The listing builds one solid part. Answer for the finished solid, in the listing's coordinates (mm). Face numbers are marked on the shaded views. A direction names the side the tool comes from. Give positions to 0.01 mm unless a question says otherwise; leave off trailing zeros. Write each loop counter-clockwise with the first axis right and the second up, starting at its lowest first coordinate (ties: lowest second). Pieces come first, ordered by that corner, then holes.
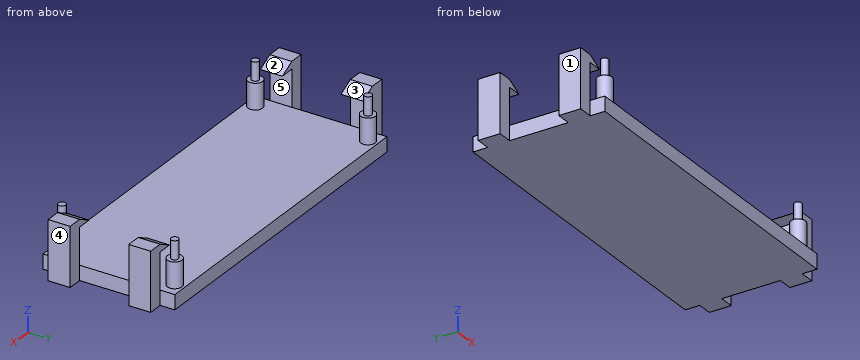
```python
from build123d import *

# Parameters (mm, degrees)
F0_R     = 1
F0_R_2   = 0.5
F1_DEPTH = 2
F2_DEPTH = 5.5
F3_DEPTH = 8
F0_W     = 2
F0_H     = 3
F4_DEPTH = 8
F6_DEPTH = 3


# Not quite as in the source:
# - a feature names something its author has since deleted; it is built from what else it names


with BuildPart() as f1:
    # F0 (on Top) → F1 (new body)
    with BuildSketch(Plane.XY):
        Polygon((22.5, 9), (-22.5, 9), (-22.5, 7), (-22.5, 4), (-22.5, -4), (-22.5, -7), (-22.5, -9), (22.5, -9), (22.5, -7), (22.5, -4), (22.5, 4), (22.5, 7), align=None)
        with Locations((-20.5, -7.7)):
            Circle(F0_R, mode=Mode.SUBTRACT)
        with Locations((20.5, -7.7)):
            Circle(F0_R, mode=Mode.SUBTRACT)
        with Locations((-20.5, 7.7)):
            Circle(F0_R, mode=Mode.SUBTRACT)
        with Locations((20.5, 7.7)):
            Circle(F0_R, mode=Mode.SUBTRACT)
        with Locations((-20.5, 7.7)):
            Circle(F0_R)
        with Locations((-20.5, 7.7)):
            Circle(F0_R_2, mode=Mode.SUBTRACT)
        with Locations((20.5, 7.7)):
            Circle(F0_R)
        with Locations((20.5, 7.7)):
            Circle(F0_R_2, mode=Mode.SUBTRACT)
        with Locations((20.5, -7.7)):
            Circle(F0_R)
        with Locations((20.5, -7.7)):
            Circle(F0_R_2, mode=Mode.SUBTRACT)
        with Locations((-20.5, -7.7)):
            Circle(F0_R)
        with Locations((-20.5, -7.7)):
            Circle(F0_R_2, mode=Mode.SUBTRACT)
        with Locations((-20.5, 7.7)):
            Circle(F0_R_2)
        with Locations((20.5, 7.7)):
            Circle(F0_R_2)
        with Locations((20.5, -7.7)):
            Circle(F0_R_2)
        with Locations((-20.5, -7.7)):
            Circle(F0_R_2)
    extrude(amount=F1_DEPTH)

    # F0 (on Top) → F2 (join)
    with BuildSketch(Plane.XY):
        with Locations((-20.5, 7.7)):
            Circle(F0_R)
        with Locations((-20.5, 7.7)):
            Circle(F0_R_2, mode=Mode.SUBTRACT)
        with Locations((-20.5, 7.7)):
            Circle(F0_R_2)
        with Locations((-20.5, -7.7)):
            Circle(F0_R)
        with Locations((-20.5, -7.7)):
            Circle(F0_R_2, mode=Mode.SUBTRACT)
        with Locations((-20.5, -7.7)):
            Circle(F0_R_2)
        with Locations((20.5, 7.7)):
            Circle(F0_R)
        with Locations((20.5, 7.7)):
            Circle(F0_R_2, mode=Mode.SUBTRACT)
        with Locations((20.5, 7.7)):
            Circle(F0_R_2)
        with Locations((20.5, -7.7)):
            Circle(F0_R)
        with Locations((20.5, -7.7)):
            Circle(F0_R_2, mode=Mode.SUBTRACT)
        with Locations((20.5, -7.7)):
            Circle(F0_R_2)
    extrude(amount=F2_DEPTH)

    # F0 (on Top) → F3 (join)
    with BuildSketch(Plane.XY):
        with Locations((-20.5, 7.7)):
            Circle(F0_R_2)
        with Locations((20.5, 7.7)):
            Circle(F0_R_2)
        with Locations((20.5, -7.7)):
            Circle(F0_R_2)
        with Locations((-20.5, -7.7)):
            Circle(F0_R_2)
    extrude(amount=F3_DEPTH)

    # F0 (on Top) → F4 (join)
    with BuildSketch(Plane.XY):
        with Locations((-23.5, 5.5)):
            Rectangle(F0_W, F0_H)
    extrude(amount=F4_DEPTH)

    # F5 (on face) → F6 (join, through all)
    with BuildSketch(Plane.XZ.offset(-4)):
        Polygon((-22.5, 8), (-22.5, 6.980669219), (-20.5, 6.980669219), align=None)
    extrude(amount=-F6_DEPTH)

    # F7: F1 across plane


with BuildPart() as f1_1:
    add(f1.part)
    add(f1.part.mirror(Plane.XZ))

    # F8: F1 across plane


with BuildPart() as f1_2:
    add(f1_1.part)
    add(f1_1.part.mirror(Plane.YZ))


solid = f1_2.part
```
Item 1: Which of the six approach directions +Z, -Z, +X, -X, +Y, -Y give full straight-line access (tool end or side, diameter ignored) to the marked faces 1 and 2?
Conclusion:
face 1: +Z, -Z, -X, +Y, -Y
face 2: +Z
Item 2: A cutting plane is placed at A-A, the plane y = -7.7. Give the vertices of the cut face in (x, z).
Conclusion:
outline: (-22.5, 0) - (22.5, 0) - (22.5, 2) - (21.5, 2) - (21.5, 5.5) - (21, 5.5) - (21, 8) - (20, 8) - (20, 5.5) - (19.5, 5.5) - (19.5, 2) - (-19.5, 2) - (-19.5, 5.5) - (-20, 5.5) - (-20, 8) - (-21, 8) - (-21, 5.5) - (-21.5, 5.5) - (-21.5, 2) - (-22.5, 2) - close
Item 3: A cutting plane is placed at C-C, the plane x = 16.5. Give the vertices of the cut face in (y, z), plus the area to 3 significant figures.
Conclusion:
outline: (-9, 0) - (9, 0) - (9, 2) - (-9, 2) - close
area: 36.0 mm2
Item 4: Consider probe 1 along X at (y, z) = (-6.5, 2.75); probe 2 along Z at (x, y) = (-11.5, -3); probe 3 along X at (y, z) = (-8, 5.75). Determine where each line is inside the solid, lowest interval first.
Conclusion:
probe 1: x = -24.5 to -22.5, 22.5 to 24.5
probe 2: z = 0 to 2
probe 3: x = -20.9 to -20.1, 20.1 to 20.9
Item 5: A cutting plane is placed at B-B, the plane z = 1.25. Give the vertices of the cut face in (x, y), plus the area to 3 significant figures.
Conclusion:
outline: (-24.5, -7) - (-22.5, -7) - (-22.5, -9) - (22.5, -9) - (22.5, -7) - (24.5, -7) - (24.5, -4) - (22.5, -4) - (22.5, 4) - (24.5, 4) - (24.5, 7) - (22.5, 7) - (22.5, 9) - (-22.5, 9) - (-22.5, 7) - (-24.5, 7) - (-24.5, 4) - (-22.5, 4) - (-22.5, -4) - (-24.5, -4) - close
area: 834 mm2
Item 6: A cutting plane is placed at D-D, the plane y = 6. Give the vertices of the cut face in (x, z), plus the area to 3 significant figures.
Conclusion:
outline: (-24.5, 0) - (24.5, 0) - (24.5, 8) - (22.5, 8) - (20.5, 6.98) - (22.5, 6.98) - (22.5, 2) - (-22.5, 2) - (-22.5, 6.98) - (-20.5, 6.98) - (-22.5, 8) - (-24.5, 8) - close
area: 124 mm2
Item 7: Each of these flat-tipped pins is pushed along its axis until it touches: P1, Ø10, axis at x = -5, y = -3, coming from the +Z side; P2, Ø1, axis at x = -21, y = 7, coming from the +Z side; P3, Ø1.2, axis at x = 22.5, z = 4, coming from the +Y side; P4, Ø1.6, axis at y = -8, z = 0.5, coming from the -X side. Where does it stop, or does it pass through?
Conclusion:
P1: stops at z = 2
P2: stops at z = 8
P3: stops at y = 7
P4: stops at x = -22.5
Item 8: Determine the mould class of the marked faces 3, 4 and 5 for opening direction Z: pulls with the +Z half, pulls with the -Z half, needs draft (parallel to the pull), parting line crosses it, or undercut.
Conclusion:
face 3: pulls with the +Z half
face 4: needs draft
face 5: undercut
